from build123d import *

# Parameters (mm, degrees)
PAD_DEPTH            = 29.25
POCKET_DEPTH         = 27.45
POCKET002_DEPTH      = 8.501
POCKET002_DEPTH_BACK = 8.501
SKETCH017_W          = 12
SKETCH017_H          = 20
POCKET003_DEPTH      = 7.5
SKETCH018_R          = 1.15
POCKET004_DEPTH      = 1.801
POCKET004_DEPTH_BACK = 14.201


with BuildPart() as part:
    # Sketch → Pad (new body, symmetric)
    with BuildSketch(Plane.XZ):
        with BuildLine():
            Line((-3.5, 14.2), (3.5, 14.2))
            ThreePointArc((8.5, 9.2), (7.035534, 12.735534), (3.5, 14.2))
            Line((8.5, 9.2), (8.5, -1.8))
            Line((8.5, -1.8), (-8.5, -1.8))
            Line((-8.5, -1.8), (-8.5, 9.2))
            ThreePointArc((-3.5, 14.2), (-7.035534, 12.735534), (-8.5, 9.2))
        make_face()
    extrude(amount=PAD_DEPTH, both=True)

    # Sketch014 → Pocket (cut, symmetric)
    with BuildSketch(Plane.XZ):
        with BuildLine():
            Line((-7.5, 0), (7.5, 0))
            Line((7.5, 0), (7.5, 9))
            ThreePointArc((7.5, 9), (6.328427, 11.828427), (3.5, 13))
            Line((3.5, 13), (-3.5, 13))
            ThreePointArc((-3.5, 13), (-6.328427, 11.828427), (-7.5, 9))
            Line((-7.5, 9), (-7.5, 0))
        make_face()
    extrude(amount=POCKET_DEPTH, both=True, mode=Mode.SUBTRACT)

    # Sketch016 → Pocket002 (cut, two sides)
    with BuildSketch(Plane.YZ) as pocket002_sk:
        with BuildLine():
            Line((-5.5, 12.7), (5.5, 12.7))
            ThreePointArc((7.5, 10.7), (6.914214, 12.114214), (5.5, 12.7))
            Line((7.5, 10.7), (7.5, 7.2))
            ThreePointArc((7.5, 7.2), (7.792893, 6.492893), (8.5, 6.2))
            Line((8.5, 6.2), (26.45, 6.2))
            ThreePointArc((26.45, 6.2), (27.157107, 6.492893), (27.45, 7.2))
            Line((27.45, 22.7), (27.45, 7.2))
            Line((-27.45, 22.7), (27.45, 22.7))
            Line((-27.45, 7.2), (-27.45, 22.7))
            ThreePointArc((-27.45, 7.2), (-27.157107, 6.492893), (-26.45, 6.2))
            Line((-8.5, 6.2), (-26.45, 6.2))
            ThreePointArc((-8.5, 6.2), (-7.792893, 6.492893), (-7.5, 7.2))
            Line((-7.5, 10.7), (-7.5, 7.2))
            ThreePointArc((-5.5, 12.7), (-6.914214, 12.114214), (-7.5, 10.7))
        make_face()
    extrude(amount=-POCKET002_DEPTH, mode=Mode.SUBTRACT)
    extrude(pocket002_sk.sketch, amount=POCKET002_DEPTH_BACK, mode=Mode.SUBTRACT)

    # Sketch017 → Pocket003 (cut, symmetric)
    with BuildSketch(Plane.XZ):
        with Locations((0, 11)):
            Rectangle(SKETCH017_W, SKETCH017_H)
    extrude(amount=POCKET003_DEPTH, both=True, mode=Mode.SUBTRACT)

    # Sketch018 → Pocket004 (cut, two sides)
    with BuildSketch(Plane.XY) as pocket004_sk:
        with Locations((-6.05, 24.25)):
            Circle(SKETCH018_R)
        with Locations((6.05, -24.25)):
            Circle(SKETCH018_R)
    extrude(amount=-POCKET004_DEPTH, mode=Mode.SUBTRACT)
    extrude(pocket004_sk.sketch, amount=POCKET004_DEPTH_BACK, mode=Mode.SUBTRACT)


solid = part.part
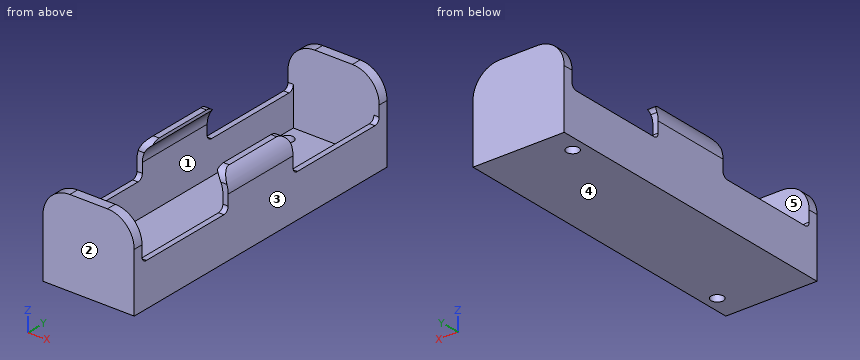
Model file for the job. Use its own axes, mm. Face numbers are marked on the shaded views. A direction names the side the tool comes from. Give positions to 0.01 mm unless a question says otherwise; leave off trailing zeros. Write each loop counter-clockwise with the first axis right and the second up, starting at its lowest first coordinate (ties: lowest second). Pieces come first, ordered by that corner, then holes. Notation, with made-up numbers: (36.5, 16.5) - (77.5, 16.5) arc R4 ccw to (77.5, 23.5) - close; hole circle Ø7 at (82.25, 78.25). An arc over 180 degrees is marked (long way). Answer as CSV lines item,"result".
1. 3-axis set-ups, long thin cutter, end or side, ignore diameter. For the marked faces 4 and 5: which of +Z, -Z, +X, -X, +Y, -Y reach the whole face in a straight line?
Responses:
face 4,"-Z, +X, -X, +Y, -Y"
face 5,"+Z"
2. Band-saw the part on D-D (y = -12). Write the cut outline in (x, z).
Responses:
outline,"(-8.5, -1.8) - (8.5, -1.8) - (8.5, 6.2) - (7.5, 6.2) - (7.5, 0) - (-7.5, 0) - (-7.5, 6.2) - (-8.5, 6.2) - close"
3. Two-plate mould, pull along X, no slides. Class the marked faces 1, 2 and 3: +X half, -X half, draft (parallel to the pull), parting line (faces both ways), or undercut.
Responses:
face 1,"undercut"
face 2,"draft"
face 3,"+X half"
4. Band-saw the part on C-C (x = 2.25). Write the cut outline in (y, z), and give its area (3 significant figures).
Responses:
outline,"(-29.25, -1.8) - (29.25, -1.8) - (29.25, 14.2) - (27.45, 14.2) - (27.45, 0) - (-27.45, 0) - (-27.45, 14.2) - (-29.25, 14.2) - close"
area,"156 mm2"
5. Pin check, flat tips, straight feed: pin 1 (0.9 mm diameter, centred on x = 6.5, y = 2.5, fed in from +Z); pin 2 (2.5 mm diameter, centred on x = -6.05, y = 24.25, fed in from -Z); pin 3 (4.5 mm diameter, centred on x = 2, y = -6.5, fed in from +Z); pin 4 (0.5 mm diameter, centred on x = -8, y = 17, fed in from +Z). Stop position of each tip, or through.
Responses:
pin 1,"stops at z = 12.7"
pin 2,"stops at z = -1.8"
pin 3,"stops at z = 0"
pin 4,"stops at z = 6.2"
6. Drill centre lines: L1, parallel to Y at x = -7.5, z = 10.25; L2, parallel to Y at x = -6.25, z = 8.5; L3, parallel to Y at x = -6.05, z = -1.05. Where is each one in solid material? Low to high. Write a range as [from, to].
Responses:
L1,"y = [-29.25, -27.45], [-7.5, 7.5], [27.45, 29.25]"
L2,"y = [-29.25, -27.45], [27.45, 29.25]"
L3,"y = [-29.25, 23.1], [25.4, 29.25]"
7. Band-saw the part on A-A (z = 1.5). Write the cut outline in (x, y).
Responses:
outline,"(-8.5, -29.25) - (8.5, -29.25) - (8.5, 29.25) - (-8.5, 29.25) - close; hole (-7.5, -27.45) - (7.5, -27.45) - (7.5, 27.45) - (-7.5, 27.45) - close"
8. Band-saw the part on B-B (y = -24.25). Write the cut outline in (x, z).
Responses:
outline,"(-8.5, -1.8) - (4.9, -1.8) - (4.9, 0) - (-7.5, 0) - (-7.5, 6.2) - (-8.5, 6.2) - close; (7.2, -1.8) - (8.5, -1.8) - (8.5, 6.2) - (7.5, 6.2) - (7.5, 0) - (7.2, 0) - close"
